The listing builds one solid part. Answer for the finished solid, in the listing's coordinates (mm). A direction names the side the tool comes from. Give positions to 0.01 mm unless a question says otherwise; leave off trailing zeros. Write each loop counter-clockwise with the first axis right and the second up, starting at its lowest first coordinate (ties: lowest second). Pieces come first, ordered by that corner, then holes. Notation, with made-up numbers: (74, -37.5) - (90, -37.5) arc R24 ccw to (90, -13.5) - close; hole circle Ø9 at (-4, -22). An arc over 180 degrees is marked (long way). One line per question, with ' | ' between items. Start each with the question number.
1. A cutting plane is placed at A-A (y = -0.5). Determine the outline of the cut face in (x, z).
2. A cutting plane is placed at C-C (x = -3). Determine the outline of the cut face in (y, z), then the cut area to 3 significant figures.
3. Given P1, Ø0.9, axis at x = 3, y = 0, coming from the +Z side; P2, Ø1.5, axis at y = 0.5, z = 8.5, coming from the -X side, each flat-ended and moving along its own axis, determine where each tip first touches the part or whether it passes through.
4. For faces 1 (the face through (-3, 0, 7.5)), 2 (the face through (2, 0, 9)), 3 (the face through (0, 0, -10.5)), determine the directions among +Z, -Z, +X, -X, +Y, -Y from which every point of the face is accessible in a straight line to the end or side of a thin tool.
5. Find the intervals of material crossed by L1, parallel to X at y = -1.2, z = 9; L2, parallel to Z at x = -2.5, y = -0.4; L3, parallel to X at y = -1.1, z = -9, in increasing order. Write a range as from..to.
6. A cutting plane is placed at B-B (z = -8.5). Determine the outline of the cut face in (x, y), then the cut area to 3 significant figures.
```python
from build123d import *

# Parameters (mm, degrees)
BOSS_EXTRUDE4_DEPTH = 1.5
SKETCH8_W           = 4
SKETCH8_H           = 3
BOSS_EXTRUDE5_DEPTH = 1.5


with BuildPart() as part:
    # Sketch6 → Boss-Extrude4 (new body, symmetric)
    with BuildSketch(Plane(origin=(0, 0, 0), x_dir=(1, 0, 0), z_dir=(0, 1, 0))):
        with BuildLine():
            Line((-2, 10.5), (2, 10.5))
            ThreePointArc((2, 10.5), (4.121320344, 9.621320344), (5, 7.5))
            Line((5, 7.5), (5, -7.5))
            Line((5, -7.5), (-5, -7.5))
            Line((-5, -7.5), (-5, 7.5))
            ThreePointArc((-5, 7.5), (-4.121320344, 9.621320344), (-2, 10.5))
        make_face()
    extrude(amount=BOSS_EXTRUDE4_DEPTH, both=True)

    # Sketch8 → Boss-Extrude5 (add, symmetric)
    with BuildSketch(Plane(origin=(0, 0, 0), x_dir=(1, 0, 0), z_dir=(0, 1, 0))):
        with Locations((0, -9)):
            Rectangle(SKETCH8_W, SKETCH8_H)
    extrude(amount=BOSS_EXTRUDE5_DEPTH, both=True)


solid = part.part
```
Determined:
1) outline: (-5, -7.5) arc R3 ccw to (-2, -10.5) - (2, -10.5) arc R3 ccw to (5, -7.5) - (5, 7.5) - (2, 7.5) - (2, 10.5) - (-2, 10.5) - (-2, 7.5) - (-5, 7.5) - close
2) outline: (-1.5, -10.33) - (1.5, -10.33) - (1.5, 7.5) - (-1.5, 7.5) - close | area: 53.5 mm2
3) P1: z = 7.5 | P2: x = -2
4) face 1: +Z, -X, +Y, -Y | face 2: +Z, +X, +Y, -Y | face 3: -Z, +X, -X, +Y, -Y
5) L1: -2..2 | L2: -10.46..7.5 | L3: -4.6..4.6
6) outline: (-4.83, -1.5) - (4.83, -1.5) - (4.83, 1.5) - (-4.83, 1.5) - close | area: 29.0 mm2
